Here's how the part is built. I have some questions about the finished solid (model axes, mm). Coordinates: 2 decimals unless noted, no trailing zeros. Order: outer loops, then holes, each group sorted by start corner. A loop starts at its lowest first (then second) coordinate and runs counter-clockwise, first axis right, second up.
```python
from build123d import *

# Parameters (mm, degrees)
F4_DEPTH = 19.05


# Not quite as in the source:
# - a length typed as a fraction of an inch, garbled in the dataset ("3 / 203.2 mm" for 3/8 in), is restored


with BuildPart() as f1:
    # F0 (on Front) → F1 (revolve)
    with BuildSketch(Plane.XZ):
        with BuildLine():
            Line((-754, 0), (-750, 0))
            ThreePointArc((-750, 0), (-676.7766952966, 176.7766952966), (-500, 250))
            Line((-500, 250), (0, 250))
            Line((0, 250), (500, 250))
            ThreePointArc((500, 250), (676.7766952966, 176.7766952966), (750, 0))
            Line((750, 0), (754, 0))
            ThreePointArc((754, 0), (679.6051224214, 179.6051224214), (500, 254))
            Line((500, 254), (0, 254))
            Line((0, 254), (-500, 254))
            ThreePointArc((-500, 254), (-679.6051224214, 179.6051224214), (-754, 0))
        make_face()
    revolve(axis=Axis((-250, 0, 0), (-1, 0, 0)))

    # F3 (on offset) → F4 (join)
    with BuildSketch(Plane.YZ.offset(300)):
        with BuildLine():
            ThreePointArc((200, -156.5758602084), (0, -254), (-200, -156.5758602084))
            Line((-200, -156.5758602084), (-200, -400))
            Line((-200, -400), (200, -400))
            Line((200, -400), (200, -156.5758602084))
        make_face()
    extrude(amount=F4_DEPTH)

    # F5: F1 across plane


with BuildPart() as f1_1:
    add(f1.part)
    add(f1.part.mirror(Plane.YZ))


solid = f1_1.part
```
Q1. I need wall thicknesses on L1, parallel to Y at x = -164, z = 0; L2, parallel to X at y = -145.5, z = -371.5; L3, parallel to Z at x = -76.5, y = -165. Which ranges of each line are inside material? Lowest first, please.
Q2. Will these pins go through, and if not, where does the flat tip stop? pin 1 (3 mm diameter, centred on x = 192, z = -71.5, fed in from -Y); pin 2 (21 mm diameter, centred on x = -310.5, z = -337, fed in from +Y); pin 3 (15 mm diameter, centred on x = -309, z = -240, fed in from -Y).
Q3. If we section it at C-C on y = 0: Write out the boundary of the cut face in (x, z).
Q4. If we section it at D-D on x = 437: Write out the boundary of the cut face in (y, z).
Q5. We'd pull the mould along Y, two halves only. Please class faces 1 (the cylindrical face through (-7, -247.96, -55.06)), 2 (the flat face through (300, -3, -304)), 3 (the cylindrical face through (7, 10.99, -249.76)): pulls with the +Y half, pulls with the -Y half, needs draft (parallel to the pull), parting line crosses it, or undercut.
Q6. If we section it at B-B on z = -358: Write out the boundary of the cut face in (x, y).
Q7. If we section it at A-A on z = 0: Write out the boundary of the cut face in (x, y).
Reply:
1. L1: y = -254 to -250, 250 to 254
1. L2: x = -319.05 to -300, 300 to 319.05
1. L3: z = -193.11 to -187.82, 187.82 to 193.11
2. pin 1: stops at y = -244.16
2. pin 2: stops at y = 200
2. pin 3: stops at y = -200
3. outline: (-500, -254) - (-319.05, -254) - (-319.05, -400) - (-300, -400) - (-300, -254) - (300, -254) - (300, -400) - (319.05, -400) - (319.05, -254) - (500, -254) arc R254 ccw to (500, 254) - (-500, 254) arc R254 ccw to start; hole (-500, -250) - (500, -250) arc R250 ccw to (500, 250) - (-500, 250) arc R250 ccw to start
4. outline: circle Ø508 at (0, 0); hole circle Ø500 at (0, 0)
5. face 1: parting line crosses it
5. face 2: needs draft
5. face 3: undercut
6. outline: (-319.05, -200) - (-300, -200) - (-300, 200) - (-319.05, 200) - close; (300, -200) - (319.05, -200) - (319.05, 200) - (300, 200) - close
7. outline: (-500, -254) - (500, -254) arc R254 ccw to (500, 254) - (-500, 254) arc R254 ccw to start; hole (-500, -250) - (500, -250) arc R250 ccw to (500, 250) - (-500, 250) arc R250 ccw to start
